Could you check a few things on this model? Use its own coordinates, in mm. A direction names the side the tool comes from. Round coordinates to 2 decimals unless told otherwise and drop trailing zeros. Loops run counter-clockwise (first coordinate to the right, second up) from the corner with the lowest first, then second, coordinate; pieces in that order, holes last. Notation, with made-up numbers: (10.5, 29.25) -> (67.5, 29.25) arc R18 cw to (67.5, 63.25) -> close; hole circle Ø10 at (-27, 58). An arc over 180 degrees is marked (long way). One line per item, written item: value.
```python
from build123d import *

# Parameters (mm, degrees)
BOSS_EXTRUDE1_DEPTH = 600
SKETCH2_W           = 450
SKETCH2_H           = 140
SKETCH2_W_2         = 146.91343935
SKETCH2_H_2         = 13.581682478
SKETCH2_H_3         = 245
SKETCH2_W_3         = 443.204970856
SKETCH2_H_4         = 681.963540889
SKETCH2_W_4         = 44.98901636
SKETCH2_H_5         = 21.550878859
BOSS_EXTRUDE2_DEPTH = 10


with BuildPart() as part:
    # Sketch1 → Boss-Extrude1 (new body)
    with BuildSketch(Plane(origin=(0, 0, 0), x_dir=(1, 0, 0), z_dir=(0, 1, 0))):
        Polygon((0, 0), (0, 740), (1900, 740), (1900, 0), (1400, 0), (1400, 702.263165655), (500, 702.263165655), (500, 0), align=None)
    extrude(amount=BOSS_EXTRUDE1_DEPTH)

    # Sketch2 → Boss-Extrude2 (add)
    with BuildSketch(Plane(origin=(0, 600, 0), x_dir=(1, 0, 0), z_dir=(0, 1, 0))):
        with Locations((250.001274905, 620)):
            Rectangle(SKETCH2_W, SKETCH2_H)
        with Locations((253.905576666, 663.689083521)):
            Rectangle(SKETCH2_W_2, SKETCH2_H_2, mode=Mode.SUBTRACT)
        with Locations((250.001274905, 474.789512045)):
            Rectangle(SKETCH2_W, SKETCH2_H)
        with Locations((253.905576666, 493.689083521)):
            Rectangle(SKETCH2_W_2, SKETCH2_H_2, mode=Mode.SUBTRACT)
        with Locations((250.001274905, 328.246947066)):
            Rectangle(SKETCH2_W, SKETCH2_H)
        with Locations((253.905576666, 323.689083521)):
            Rectangle(SKETCH2_W_2, SKETCH2_H_2, mode=Mode.SUBTRACT)
        with Locations((250.001274905, 130.536459111)):
            Rectangle(SKETCH2_W, SKETCH2_H_3)
        with Locations((253.905576666, 153.689083521)):
            Rectangle(SKETCH2_W_2, SKETCH2_H_2, mode=Mode.SUBTRACT)
        with Locations((1655.213820174, 349.018229555)):
            Rectangle(SKETCH2_W_3, SKETCH2_H_4)
        with Locations((1480.203434269, 339.22456057)):
            Rectangle(SKETCH2_W_4, SKETCH2_H_5, mode=Mode.SUBTRACT)
    extrude(amount=BOSS_EXTRUDE2_DEPTH)


solid = part.part
```
(1) Imagine slicing it at B-B on x = 967. Write out the boundary of the cut face in (y, z).
Results below:
outline: (0, -740) -> (600, -740) -> (600, -702.26) -> (0, -702.26) -> close
(2) We'd pull the mould along X, two halves only. Please class faces 1 (the face through (1400, 296, -346)), 2 (the face through (1900, 296, -375)), 3 (the face through (1652, 610, -354)): +X half, -X half, draft (parallel to the pull), parting line (faces both ways), or undercut.
Results below:
face 1: undercut
face 2: +X half
face 3: draft
(3) Imagine slicing it at A-A on y = 369.5. Write out the boundary of the cut face in (x, z), then the cut area to 3 significant figures.
Results below:
outline: (0, -740) -> (1900, -740) -> (1900, 0) -> (1400, 0) -> (1400, -702.26) -> (500, -702.26) -> (500, 0) -> (0, 0) -> close
area: 774,000 mm²
(4) Please list where these lines run through material, in increasing order: L1, parallel to X at y = 31, z = -605; L2, parallel to Z at x = 684, y = 444; L3, parallel to Y at x = 491.5, z = -85.5.
Results below:
L1: x = 0 to 500, 1400 to 1900
L2: z = -740 to -702.26
L3: y = 0 to 600
(5) On a 3-axis mill with a long thin cutter (end or side, diameter ignored), from which of +Z, -Z, +X, -X, +Y, -Y can I reach the whole of each face in a straight line? I mean faces 4 (the face through (253, 296, 0)), 5 (the face through (956, 296, -702.263)). Say none if no direction works.
Results below:
face 4: +Z, +X, -X, +Y, -Y
face 5: +Z, +Y, -Y
(6) For pin 1 Ø5 at (x, y) = (275, 603) entering from +Z; pin 2 Ø5 at (y, z) = (605, -484) entering from -X; pin 3 Ø3 at (x, y) = (161, 607) entering from -Z, each with a flat end and sliding along its axis, tell me the tip position at first contact or that it passes through.
Results below:
pin 1: stops at z = -8.04
pin 2: stops at x = 25
pin 3: stops at z = -690
